Print and shaded views of the part. All mm, measured from the part's lowest x, y and z. A direction names the side the tool comes from. Give positions to 0.01 mm unless a question says otherwise; leave off trailing zeros. Write each loop counter-clockwise with the first axis right and the second up, starting at its lowest first coordinate (ties: lowest second). Pieces come first, ordered by that corner, then holes.
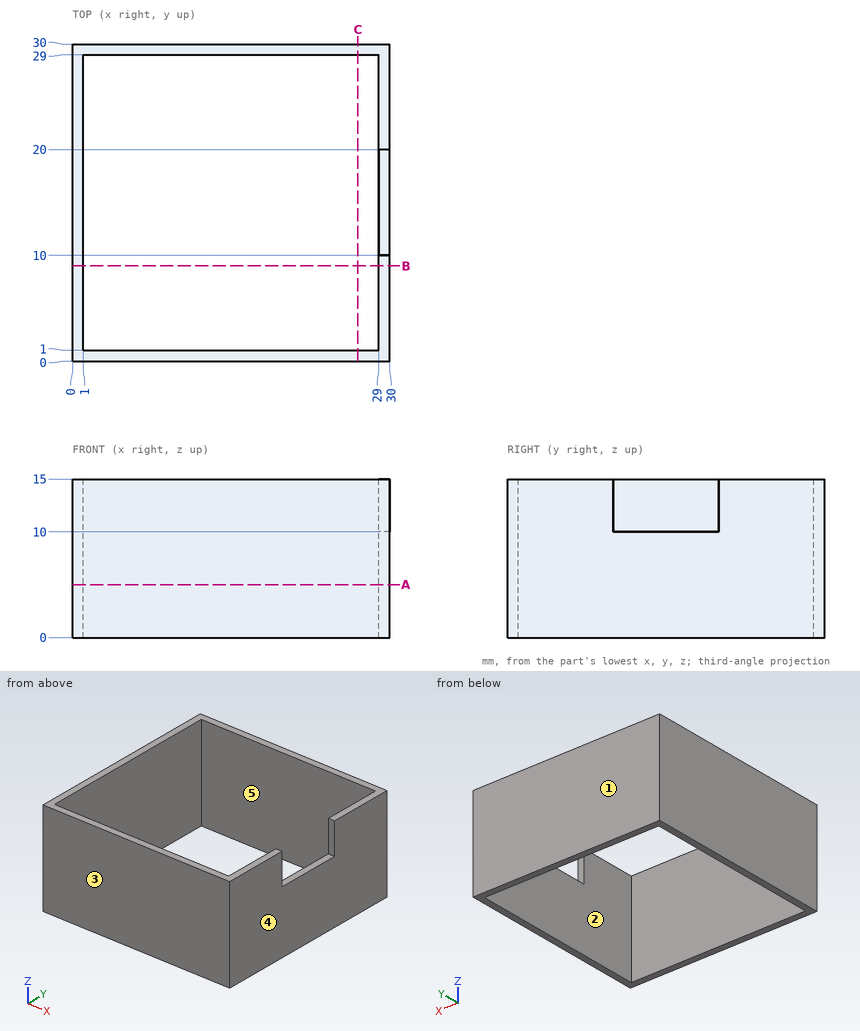
1. 3-axis set-ups, long thin cutter, end or side, ignore diameter. For the marked faces 1 and 2: which of +Z, -Z, +X, -X, +Y, -Y reach the whole face in a straight line?
2. Mould opens along X. For the marked faces 3, 4 and 5 say: pulls with the +X half, pulls with the -X half, needs draft (parallel to the pull), parting line crosses it, or undercut.
3. Drill centre lines: line 1 along X through (y, z) = (2, 6.75); line 2 along X through (y, z) = (17.5, 11.75). Where is each one in solid material? Low to high.
4. Drop a flat-ended pin along its axis: pin 1 (1.1 mm diameter, centred on x = 29.5, y = 14.5, fed in from +Z). Give the stop position or say it passes through.
5. Saw through at A-A on z = 5. Give the cut face in (x, y).
6. Saw through at B-B on y = 9. Give the cut face in (x, z).
Outcome:
1. face 1: +Z, -Z, +X, -X, +Y
1. face 2: +Z, -Z
2. face 3: needs draft
2. face 4: pulls with the +X half
2. face 5: undercut
3. line 1: x = 0 to 1, 29 to 30
3. line 2: x = 0 to 1
4. pin 1: stops at z = 10
5. outline: (0, 0) - (30, 0) - (30, 30) - (0, 30) - close; hole (1, 1) - (29, 1) - (29, 29) - (1, 29) - close
6. outline: (0, 0) - (1, 0) - (1, 15) - (0, 15) - close; (29, 0) - (30, 0) - (30, 15) - (29, 15) - close
